Geometry: final body of the model. Coordinates: model frame, mm. A direction names the side the tool comes from. Round coordinates to 2 decimals unless told otherwise and drop trailing zeros. Write each loop counter-clockwise with the first axis right and the second up, starting at its lowest first coordinate (ties: lowest second). Pieces come first, ordered by that corner, then holes. Notation, with made-up numbers: M -35.5,80 L -19.5,80 A20 cw -19.5,93 Z; hole C -17.5,72.5 d5. An arc over 180 degrees is marked long. Answer as CSV lines item,"result". Start each with the question number.
Q1. Mould query, pull axis X, two halves, no side actions, for faces 1 (the flat face through (-48.5, 5, -3)), 2 (the flat face through (38.5, 5, 7)), 3 (the flat face through (-1.58, 4.93, -117.05)). Classes: pulls with the +X half, pulls with the -X half, needs draft (parallel to the pull), parting line crosses it, or undercut.
Q2. Section query B-B on z = -7. Output: boundary loops of the cut face in (x, y).
Q3. Reachability of faces 4 (the flat face through (48.5, 5, -3)), 5 (the flat face through (-13.5, 5, -1)), 6 (the flat face through (11.601, 4.93, -100.936)), 7 (the flat face through (-25, 10, -66)) from +Z, -Z, +X, -X, +Y, -Y: full face, straight path, thin tool, end or side. Return the list, or none.
Q4. Section query D-D on z = -103. Output: boundary loops of the cut face in (x, y), and give its area (3 significant figures).
Q5. Section query C-C on x = 31.5. Output: boundary loops of the cut face in (y, z).
Q6. Ray query, probe 1 along X at (y, z) = (3.75, -3.5); probe 2 along X at (y, z) = (4.5, -111); probe 3 along X at (y, z) = (4.25, -105). Return the intervals inside material, ascending.
Q7. First-contact query: pin 1 (1 mm diameter, centred on y = 5.5, z = -25, fed in from +X); pin 2 (2 mm diameter, centred on y = 6.5, z = 7.5, fed in from -X); pin 3 (5 mm diameter, centred on x = -9.5, z = -15, fed in from +Y) (3 decimals); pin 4 (4 mm diameter, centred on x = 21, y = 1, fed in from -Z). Flat tips, straight axial feed; report the tip coordinate or a pass-through.
Q8. Section query A-A on y = 8.25. Output: boundary loops of the cut face in (x, z), and give its area (3 significant figures).
```python
from build123d import *

# Parameters (mm, degrees)
BOSS_EXTRUDE1_DEPTH = 10


with BuildPart() as part:
    # Sketch1 → Boss-Extrude1 (new body)
    with BuildSketch(Plane(origin=(0, 0, 0), x_dir=(1, 0, 0), z_dir=(0, 1, 0))):
        Polygon((13.5, 3.125985755), (13.5, -3.125985755), (13.5, -10.128193845), (23.5, -10.128193845), (23.5, -3.125985755), (38.5, -3.125985755), (38.5, -10.128193845), (48.5, -10.128193845), (48.5, -3.125985755), (48.5, 15.603410537), (94.082583098, 65.745372538), (118.364573122, 57.800903455), (121.474127931, 67.305148238), (-128.125479481, 168.208510016), (-131.873415704, 158.937427336), (-48.5, 15.603410537), (-48.5, -3.125985755), (-48.5, -10.128193845), (-38.5, -10.128193845), (-38.5, -3.125985755), (-23.5, -3.125985755), (-23.5, -10.128193845), (-13.5, -10.128193845), (-13.5, -3.125985755), (-13.5, 3.125985755), (-13.5, 13.214699594), (-24.737103286, 115.626405321), (48.971306344, 85.828977352), (13.5, 13.214699594), align=None)
        Polygon((-98.688732225, 145.522157347), (-48.5, 125.232815319), (-48.5, 57.36957732), (-100.110149338, 146.096780708), align=None, mode=Mode.SUBTRACT)
    extrude(amount=BOSS_EXTRUDE1_DEPTH)


solid = part.part
```
Entries:
1,face 1,"pulls with the -X half"
1,face 2,"undercut"
1,face 3,"pulls with the +X half"
2,outline,"M -48.5,0 L -13.5,0 L -13.5,10 L -48.5,10 Z; M 13.5,0 L 48.5,0 L 48.5,10 L 13.5,10 Z"
3,face 4,"+Z, +X, +Y, -Y"
3,face 5,"+Z, +Y, -Y"
3,face 6,"+Y, -Y"
3,face 7,"+Z, -Z, +X, -X, +Y"
4,outline,"M -99.34,0 L -75.04,0 L -75.04,10 L -99.34,10 Z; M -48.5,0 L -23.35,0 L -23.35,10 L -48.5,10 Z; M 6.5,0 L 33.18,0 L 33.18,10 L 6.5,10 Z"
4,area,"761 mm^2"
5,outline,"M 0,-103.68 L 10,-103.68 L 10,-92.89 L 0,-92.89 Z; M 0,-50.06 L 10,-50.06 L 10,3.13 L 0,3.13 Z"
6,probe 1,"x = -48.5 to -13.5, 13.5 to 48.5"
6,probe 2,"x = -103.99 to -79.7, -48.5 to -24.23, -13.29 to 13.39"
6,probe 3,"x = -100.5 to -76.21, -48.5 to -23.57, 1.55 to 28.23"
7,pin 1,"stops at x = 57.5"
7,pin 2,"stops at x = -48.5"
7,pin 3,"passes through"
7,pin 4,"stops at z = -108.73"
8,outline,"M -131.87,-158.94 L -128.13,-168.21 L 121.47,-67.31 L 118.36,-57.8 L 94.08,-65.75 L 48.5,-15.6 L 48.5,10.13 L 38.5,10.13 L 38.5,3.13 L 23.5,3.13 L 23.5,10.13 L 13.5,10.13 L 13.5,-13.21 L 48.97,-85.83 L -24.74,-115.63 L -13.5,-13.21 L -13.5,10.13 L -23.5,10.13 L -23.5,3.13 L -38.5,3.13 L -38.5,10.13 L -48.5,10.13 L -48.5,-15.6 Z; hole M -100.11,-146.1 L -48.5,-125.23 L -48.5,-57.37 Z"
8,area,"13,000 mm^2"
